```python
from build123d import *

# Parameters (mm, degrees)
F0_W     = 76.2
F0_H     = 19.05
F1_DEPTH = 1.5875
F2_R     = 1.984375
F2_R_2   = 1.9812
F3_DEPTH = 3.175
F4_DEPTH = 3.175


# Not quite as in the source:
# - a length typed as a fraction of an inch, garbled in the dataset ("3 / 203.2 mm" for 3/8 in), is restored


with BuildPart() as f1:
    # F0 (on Front) → F1 (new body, symmetric)
    with BuildSketch(Plane.XZ):
        Rectangle(F0_W, F0_H)
    extrude(amount=F1_DEPTH, both=True)

    # F2 (on face) → F3 (cut)
    with BuildSketch(Plane.XZ.offset(1.5875)):
        with Locations((6.35, 3.175)):
            Circle(F2_R)
        with Locations((6.35, -3.175)):
            Circle(F2_R_2)
        with Locations((25.4, 3.175)):
            Circle(F2_R)
        with Locations((25.4, -3.175)):
            Circle(F2_R_2)
    extrude(amount=-F3_DEPTH, mode=Mode.SUBTRACT)

    # F2 (on face) → F4 (cut)
    with BuildSketch(Plane.XZ.offset(1.5875)):
        with Locations((6.35, 3.175)):
            Circle(F2_R)
        with Locations((6.35, -3.175)):
            Circle(F2_R_2)
        with Locations((25.4, 3.175)):
            Circle(F2_R)
        with Locations((25.4, -3.175)):
            Circle(F2_R_2)
    extrude(amount=-F4_DEPTH, mode=Mode.SUBTRACT)


solid = f1.part
```
Design review of the part built by this model. Coordinates are the model's own, in mm. Coordinates: 2 decimals unless noted, no trailing zeros. Order: outer loops, then holes, each group sorted by start corner. A loop starts at its lowest first (then second) coordinate and runs counter-clockwise, first axis right, second up.
1) Wall thickness on line 1 along Z through (x, y) = (25.4, 0.3) (3 decimals): over which ranges is the line inside the solid? List them lowest first.
2) Take a section at A-A, the plane x = 25.4. Give the boundary of the cut face in (y, z) (1 decimal), and give its area (3 significant figures).
3) Mouldability with a two-part tool opening along Z and no side actions: class faces 1 (the cylindrical face through (8.18, -0.02, -3.93)), 2 (the flat face through (-1, 1.588, 0)), 3 (the flat face through (-1, 0, -9.525)) as +Z half, -Z half, draft (parallel to the pull), parting line (faces both ways), or undercut.
4) Take a section at B-B, the plane y = -0.8. Give the boundary of the cut face in (x, z) (3 decimals).
5) Clearance check with a flat-ended pin moving along its axis: pin 1 (3.5 mm diameter, centred on x = 6.35, z = 3.175, fed in from +Y). State where the tip first meets the part, or that it passes through.
Returned:
1. line 1: z = -9.525 to -5.156, -1.194 to 1.191, 5.159 to 9.525
2. outline: (-1.6, -9.5) - (1.6, -9.5) - (1.6, -5.2) - (-1.6, -5.2) - close; (-1.6, -1.2) - (1.6, -1.2) - (1.6, 1.2) - (-1.6, 1.2) - close; (-1.6, 5.2) - (1.6, 5.2) - (1.6, 9.5) - (-1.6, 9.5) - close
2. area: 35.3 mm2
3. face 1: undercut
3. face 2: draft
3. face 3: -Z half
4. outline: (-38.1, -9.525) - (38.1, -9.525) - (38.1, 9.525) - (-38.1, 9.525) - close; hole circle Ø3.969 at (6.35, 3.175); hole circle Ø3.962 at (6.35, -3.175); hole circle Ø3.969 at (25.4, 3.175); hole circle Ø3.962 at (25.4, -3.175)
5. pin 1: passes through
